Here's how the part is built. I have some questions about the finished solid (model axes, mm). A direction names the side the tool comes from. Give positions to 0.01 mm unless a question says otherwise; leave off trailing zeros. Loops run counter-clockwise (first coordinate to the right, second up) from the corner with the lowest first, then second, coordinate; pieces in that order, holes last. Notation, with made-up numbers: (76.5, -7.5) - (133.5, -7.5) arc R13 cw to (133.5, 6.5) - close; hole circle Ø5 at (29.5, 49.5). An arc over 180 degrees is marked (long way). Use one line per item in the form item = value.
from build123d import *

# Parameters (mm, degrees)
SKETCH1_R           = 12
SKETCH1_R_2         = 4
BOSS_EXTRUDE1_DEPTH = 5
CHAMFER1_SIZE       = 1


with BuildPart() as part:
    # Sketch1 → Boss-Extrude1 (new body)
    with BuildSketch(Plane(origin=(0, 0, 0), x_dir=(0, 1, 0), z_dir=(0, 0, 1))):
        with BuildLine():
            Line((6.575458392, 16.755994358), (37, 11))
            ThreePointArc((37, 11), (48, 0), (37, -11))
            Line((37, -11), (6.575458392, -16.755994358))
            ThreePointArc((6.575458392, -16.755994358), (0, -18), (-6.575458392, -16.755994358))
            Line((-6.575458392, -16.755994358), (-37, -11))
            ThreePointArc((-37, -11), (-48, 0), (-37, 11))
            Line((-37, 11), (-6.575458392, 16.755994358))
            ThreePointArc((-6.575458392, 16.755994358), (0, 18), (6.575458392, 16.755994358))
        make_face()
        with Locations(Location((0, 0, 0), (0, 0, 270))):
            Circle(SKETCH1_R, mode=Mode.SUBTRACT)
        with Locations(Location((37, 0, 0), (0, 0, 270))):
            Circle(SKETCH1_R_2, mode=Mode.SUBTRACT)
        with Locations(Location((-37, 0, 0), (0, 0, 90))):
            Circle(SKETCH1_R_2, mode=Mode.SUBTRACT)
        with BuildLine():
            Line((23.448643014, 8.475075542), (22.218560764, 8.707793806))
            ThreePointArc((22.218560764, 8.707793806), (18.601781162, 7.560433495), (17.570449711, 3.908874128))
            ThreePointArc((17.570449711, 3.908874128), (18, 0), (17.570449711, -3.908874128))
            ThreePointArc((17.570449711, -3.908874128), (18.601781162, -7.560433495), (22.218560764, -8.707793806))
            Line((22.218560764, -8.707793806), (23.448643014, -8.475075542))
            ThreePointArc((23.448643014, -8.475075542), (26.140025122, -6.594459623), (26.517055984, -3.332849344))
            ThreePointArc((26.517055984, -3.332849344), (26, 0), (26.517055984, 3.332849344))
            ThreePointArc((26.517055984, 3.332849344), (26.140025122, 6.594459623), (23.448643014, 8.475075542))
        make_face(mode=Mode.SUBTRACT)
        with BuildLine():
            Line((-23.448643014, -8.475075542), (-22.218560764, -8.707793806))
            ThreePointArc((-22.218560764, -8.707793806), (-18.601781162, -7.560433495), (-17.570449711, -3.908874128))
            ThreePointArc((-17.570449711, -3.908874128), (-18, 0), (-17.570449711, 3.908874128))
            ThreePointArc((-17.570449711, 3.908874128), (-18.601781162, 7.560433495), (-22.218560764, 8.707793806))
            Line((-22.218560764, 8.707793806), (-23.448643014, 8.475075542))
            ThreePointArc((-23.448643014, 8.475075542), (-26.140025122, 6.594459623), (-26.517055984, 3.332849344))
            ThreePointArc((-26.517055984, 3.332849344), (-26, 0), (-26.517055984, -3.332849344))
            ThreePointArc((-26.517055984, -3.332849344), (-26.140025122, -6.594459623), (-23.448643014, -8.475075542))
        make_face(mode=Mode.SUBTRACT)
    extrude(amount=BOSS_EXTRUDE1_DEPTH)

    # Chamfer1
    chamfer1_edges = [part.edges().sort_by_distance(p)[0] for p in [
        (-4, 37, 5),
        (4, -37, 5),
    ]]
    chamfer(chamfer1_edges, length=CHAMFER1_SIZE)


solid = part.part
(1) If I drill on probe 1 along Y at (x, z) = (0, 3.95); probe 2 along X at (y, z) = (-37, 2.75); probe 3 along Y at (x, z) = (7, 3.6), over which ranges is the centre line in solid material (lowest first)?
Geometry says:
probe_1 = -48 to -41, -33 to -26, -18 to -12, 12 to 18, 26 to 33, 41 to 48
probe_2 = -11 to -4, 4 to 11
probe_3 = -45.49 to -25.86, -18.15 to -9.75, 9.75 to 18.15, 25.86 to 45.49
(2) If we section it at D-D (y = -29): List the corners of the cut face in (x, z) for me.
Geometry says:
outline = (-12.51, 0) - (12.51, 0) - (12.51, 5) - (-12.51, 5) - close
(3) For faces 4 (the flat face through (13.838, 22.001, 2.465)), 5 (the cylindrical face through (0, 26, 2)), which set-ups out of +Z, -Z, +X, -X, +Y, -Y let a thin tool reach every point of the face, with its end or its side?
Geometry says:
face_4 = +Z, -Z, +X, +Y
face_5 = +Z, -Z
(4) If we section it at C-C (x = -10): List the corners of the cut face in (y, z) for me.
Geometry says:
outline = (-41.58, 0) - (-6.63, 0) - (-6.63, 5) - (-41.58, 5) - close; (6.63, 0) - (41.58, 0) - (41.58, 5) - (6.63, 5) - close
(5) For P1, Ø10.5, axis at x = 0, y = -37, coming from the -Z side; P2, Ø9, axis at x = 0, y = 37, coming from the +Z side; P3, Ø3, axis at x = 4, z = 3.5, coming from the +Y side, each with a flat end and sliding along its axis, tell me the tip position at first contact or that it passes through.
Geometry says:
P1 = 0
P2 = 4.5
P3 = 47.71
(6) If we section it at B-B (x = 0): List the corners of the cut face in (y, z) for me.
Geometry says:
outline = (-48, 0) - (-41, 0) - (-41, 4) - (-42, 5) - (-48, 5) - close; (-33, 0) - (-26, 0) - (-26, 5) - (-32, 5) - (-33, 4) - close; (-18, 0) - (-12, 0) - (-12, 5) - (-18, 5) - close; (12, 0) - (18, 0) - (18, 5) - (12, 5) - close; (26, 0) - (33, 0) - (33, 4) - (32, 5) - (26, 5) - close; (41, 0) - (48, 0) - (48, 5) - (42, 5) - (41, 4) - close
(7) Thinking about a two-plate mould opening in Y: for faces 1 (the cylindrical face through (0, 18, 2)), 2 (the flat face through (8, 11, 0)), 3 (the cylindrical face through (0, -48, 2)), which applies, pulls with the +Y half, pulls with the -Y half, needs draft (parallel to the pull), parting line crosses it, or undercut?
Geometry says:
face_1 = undercut
face_2 = needs draft
face_3 = pulls with the -Y half
(8) If we section it at A-A (y = 0): List the corners of the cut face in (x, z) for me.
Geometry says:
outline = (-18, 0) - (-12, 0) - (-12, 5) - (-18, 5) - close; (12, 0) - (18, 0) - (18, 5) - (12, 5) - close
